from build123d import *

# Parameters (mm, degrees)
SKETCH1_R           = 4
BOSS_EXTRUDE1_DEPTH = 3
FILLET1_R           = 10


with BuildPart() as part:
    # Sketch1 → Boss-Extrude1 (new body)
    with BuildSketch(Plane.XY):
        Polygon((-60, 60), (-60, 10), (-22.5, -60), (22.5, -60), (60, 10), (60, 60), align=None)
        with Locations((-42, 40)):
            Circle(SKETCH1_R, mode=Mode.SUBTRACT)
        with Locations((0, -40)):
            Circle(SKETCH1_R, mode=Mode.SUBTRACT)
        with Locations((0, -10)):
            Circle(SKETCH1_R, mode=Mode.SUBTRACT)
        with Locations((0, 40)):
            Circle(SKETCH1_R, mode=Mode.SUBTRACT)
        with Locations(Location((42, 40, 0), (0, 0, 180))):
            Circle(SKETCH1_R, mode=Mode.SUBTRACT)
    extrude(amount=BOSS_EXTRUDE1_DEPTH)

    # Fillet1
    fillet1_edges = [part.edges().sort_by_distance(p)[0] for p in [
        (60, 60, 1.5),
        (60, 10, 1.5),
        (22.5, -60, 1.5),
        (-22.5, -60, 1.5),
        (-60, 10, 1.5),
        (-60, 60, 1.5),
    ]]
    fillet(fillet1_edges, radius=FILLET1_R)


solid = part.part
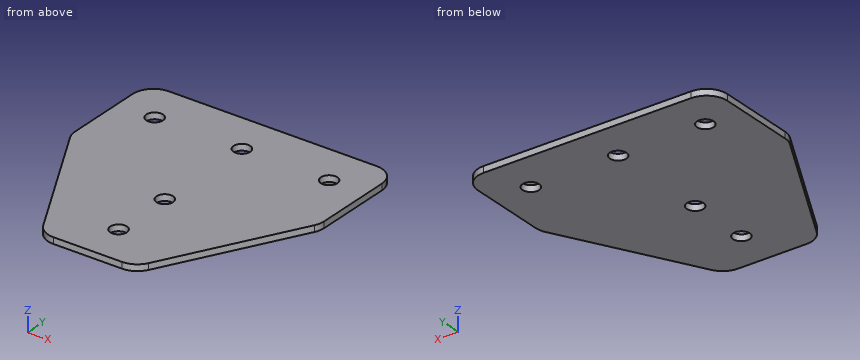
Could you check a few things on this model? Use its own coordinates, in mm. Give positions to 0.01 mm unless a question says otherwise; leave off trailing zeros. Write each loop counter-clockwise with the first axis right and the second up, starting at its lowest first coordinate (ties: lowest second). Pieces come first, ordered by that corner, then holes. Notation, with made-up numbers: (27.5, 72) -> (56.5, 72) arc R31 cw to (56.5, 108) -> close; hole circle Ø11 at (49.5, 60). An arc over 180 degrees is marked (long way). Answer as CSV lines item,"result". Start each with the question number.
(1) If we section it at C-C, the plane z = 1.3: Write out the boundary of the cut face in (x, y), and give its area (3 significant figures).
(2) If we section it at A-A, the plane x = 0: Write out the boundary of the cut face in (y, z), and give its area (3 significant figures).
(3) Please list where these lines run through material, in increasing order: line 1 (Y direction, x = 0, z = 0.6); line 2 (X direction, y = -9, z = 1.2); line 3 (X direction, y = -11, z = 1.5).
(4) I'm going to push a flat-ended pin straight in: pin 1 Ø9 at (x, y) = (42, 40) entering from -Z. Where does the tip first touch, or does it pass through?
(5) If we section it at D-D, the plane x = 42: Write out the boundary of the cut face in (y, z), and give its area (3 significant figures).
(6) If we section it at B-B, the plane y = 40: Write out the boundary of the cut face in (x, z), and give its area (3 significant figures).
Answer list:
1,outline,"(-60, 12.51) arc R10 ccw to (-58.81, 7.79) -> (-25.33, -54.72) arc R10 ccw to (-16.51, -60) -> (16.51, -60) arc R10 ccw to (25.33, -54.72) -> (58.81, 7.79) arc R10 ccw to (60, 12.51) -> (60, 50) arc R10 ccw to (50, 60) -> (-50, 60) arc R10 ccw to (-60, 50) -> close; hole circle Ø8 at (-42, 40); hole circle Ø8 at (0, -40); hole circle Ø8 at (0, -10); hole circle Ø8 at (0, 40); hole circle Ø8 at (42, 40)"
1,area,"11,500 mm^2"
2,outline,"(-60, 0) -> (-44, 0) -> (-44, 3) -> (-60, 3) -> close; (-36, 0) -> (-14, 0) -> (-14, 3) -> (-36, 3) -> close; (-6, 0) -> (36, 0) -> (36, 3) -> (-6, 3) -> close; (44, 0) -> (60, 0) -> (60, 3) -> (44, 3) -> close"
2,area,"288 mm^2"
3,line 1,"-60 to -44, -36 to -14, -6 to 36, 44 to 60"
3,line 2,"-49.82 to -3.87, 3.87 to 49.82"
3,line 3,"-48.75 to -3.87, 3.87 to 48.75"
4,pin 1,"z = 0"
5,outline,"(-23.6, 0) -> (36, 0) -> (36, 3) -> (-23.6, 3) -> close; (44, 0) -> (60, 0) -> (60, 3) -> (44, 3) -> close"
5,area,"227 mm^2"
6,outline,"(-60, 0) -> (-46, 0) -> (-46, 3) -> (-60, 3) -> close; (-38, 0) -> (-4, 0) -> (-4, 3) -> (-38, 3) -> close; (4, 0) -> (38, 0) -> (38, 3) -> (4, 3) -> close; (46, 0) -> (60, 0) -> (60, 3) -> (46, 3) -> close"
6,area,"288 mm^2"
